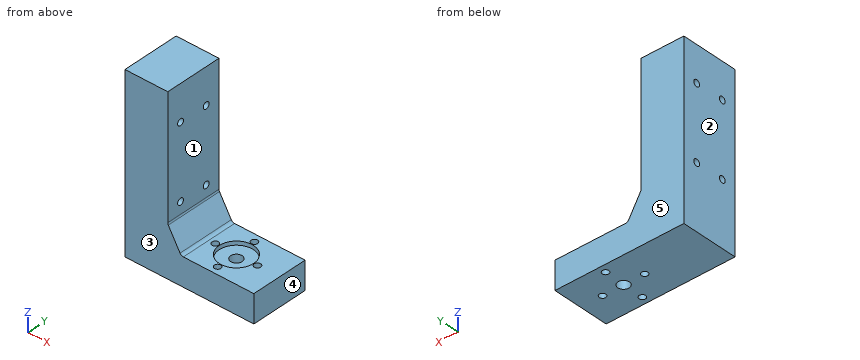
```python
from build123d import *

# Parameters (mm, degrees)
BOSS_EXTRUDE1_DEPTH = 300
SKETCH3_R           = 17
SKETCH3_R_2         = 30
CUT_EXTRUDE1_DEPTH  = 1055.907875982
SKETCH4_R           = 90
CUT_EXTRUDE2_DEPTH  = 20
SKETCH5_R           = 17
CUT_EXTRUDE3_DEPTH  = 1051
CHAMFER1_SIZE       = 70
CHAMFER1_SIZE2      = 120
FILLET1_R           = 20
SCALE1_SCALE        = 0.1


with BuildPart() as part:
    # Sketch2 → Boss-Extrude1 (new body)
    with BuildSketch(Plane(origin=(0, 0, 0), x_dir=(-1, 0, 0), z_dir=(0, 1, 0))):
        Polygon((0, 0), (673.85334868, 0), (673.85334868, 900), (450, 900), (450, 145.843324447), (0, 145.843324447), align=None)
    extrude(amount=BOSS_EXTRUDE1_DEPTH)

    # Sketch3 → Cut-Extrude1 (cut, through all)
    with BuildSketch(Plane.XY.offset(145.843324447)):
        with Locations((-335, 150)):
            Circle(SKETCH3_R)
        with Locations((-228.822978678, 259.933547355)):
            Circle(SKETCH3_R)
        with Locations((-115, 150)):
            Circle(SKETCH3_R)
        with Locations((-225, 40)):
            Circle(SKETCH3_R)
        with Locations((-225, 150)):
            Circle(SKETCH3_R_2)
    extrude(amount=-CUT_EXTRUDE1_DEPTH, mode=Mode.SUBTRACT)

    # Sketch4 → Cut-Extrude2 (cut)
    with BuildSketch(Plane.XY.offset(145.843324447)):
        with Locations((-225, 150)):
            Circle(SKETCH4_R)
    extrude(amount=-CUT_EXTRUDE2_DEPTH, mode=Mode.SUBTRACT)

    # Sketch5 → Cut-Extrude3 (cut, through all)
    with BuildSketch(Plane.YZ.offset(-450)):
        with Locations(Location((75, 713.5, 0), (0, 0, 270))):
            Circle(SKETCH5_R)
        with Locations(Location((225, 713.5, 0), (0, 0, 270))):
            Circle(SKETCH5_R)
        with Locations(Location((75, 332.343324447, 0), (0, 0, 270))):
            Circle(SKETCH5_R)
        with Locations(Location((225, 332.343324447, 0), (0, 0, 270))):
            Circle(SKETCH5_R)
    extrude(amount=-CUT_EXTRUDE3_DEPTH, mode=Mode.SUBTRACT)

    # Chamfer1
    chamfer1_edges = [part.edges().sort_by_distance(p)[0] for p in [
        (-450, 150, 145.843324447),
    ]]
    chamfer1_side = [part.faces().sort_by_distance(p)[0] for p in [
        (-444.591673087, 150, 145.843324447),
    ]]
    chamfer(chamfer1_edges, length=CHAMFER1_SIZE, length2=CHAMFER1_SIZE2, reference=chamfer1_side[0])

    # Fillet1
    fillet1_edges = [part.edges().sort_by_distance(p)[0] for p in [
        (-380, 150, 145.843324447),
        (-450, 150, 265.843324447),
    ]]
    fillet(fillet1_edges, radius=FILLET1_R)


with BuildPart() as part_1:
    # Scale1: scaled about (-481.914690358, 150.000111117, 357.549237265)
    add(part.part.scale(SCALE1_SCALE).moved(Location((-433.723221322, 135.000100005, 321.794313538))))


solid = part_1.part
```
Here's how the part is built. I have some questions about the finished solid (model axes, mm). Face numbers are marked on the shaded views. A direction names the side the tool comes from. Round coordinates to 2 decimals unless told otherwise and drop trailing zeros. Loops run counter-clockwise (first coordinate to the right, second up) from the corner with the lowest first, then second, coordinate; pieces in that order, holes last.
1. Will these pins go through, and if not, where does the flat tip stop? pin 1 (4 mm diameter, centred on y = 152, z = 387, fed in from +X); pin 2 (4 mm diameter, centred on x = -456.61, y = 160.99, fed in from -Z); pin 3 (3 mm diameter, centred on x = -445.22, y = 150, fed in from -Z); pin 4 (14.5 mm diameter, centred on x = -455.5, y = 154, fed in from +Z).
Answers:
pin 1: stops at x = -478.72
pin 2: stops at z = 321.79
pin 3: passes through
pin 4: stops at z = 336.38
2. If I drill on probe 1 along Z at (x, y) = (-441.5, 158); probe 2 along X at (y, z) = (139, 384); probe 3 along Z at (x, y) = (-451.5, 143.5), over which ranges is the centre line in solid material (lowest first)?
Answers:
probe 1: z = 321.79 to 336.38
probe 2: x = -501.11 to -478.72
probe 3: z = 321.79 to 334.38
3. Thinking about a two-plate mould opening in Y: for the marked faces 3, 4 and 5, which applies, released by +Y, released by -Y, zero draft, split by the parting line, or undercut?
Answers:
face 3: released by -Y
face 4: zero draft
face 5: released by +Y
4. Suppose I cut it at C-C, the plane z = 371. Please give me the cut outline in (x, y).
Answers:
outline: (-501.11, 135) - (-478.72, 135) - (-478.72, 165) - (-501.11, 165) - close
5. Suppose I cut it at A-A, the plane z = 332.5. Please give me the cut outline in (x, y).
Answers:
outline: (-501.11, 135) - (-433.72, 135) - (-433.72, 165) - (-501.11, 165) - close; hole circle Ø3.4 at (-467.22, 150); hole circle Ø6 at (-456.22, 150); hole circle Ø3.4 at (-456.61, 160.99); hole circle Ø3.4 at (-456.22, 139); hole circle Ø3.4 at (-445.22, 150)
6. Suppose I cut it at B-B, the plane x = -441.5. Please give me the cut outline in (y, z).
Answers:
outline: (135, 321.79) - (165, 321.79) - (165, 336.38) - (135, 336.38) - close
7. For the marked faces 1 and 2, which set-ups out of +Z, -Z, +X, -X, +Y, -Y let a thin tool reach every point of the face, with its end or its side?
Answers:
face 1: +Z, +X, +Y, -Y
face 2: +Z, -Z, -X, +Y, -Y
